Source: CAD feature listing. Evaluate the final solid. Frame: model axes, mm. A direction names the side the tool comes from. Round coordinates to 2 decimals unless told otherwise and drop trailing zeros. Write each loop counter-clockwise with the first axis right and the second up, starting at its lowest first coordinate (ties: lowest second). Pieces come first, ordered by that corner, then holes. Notation, with made-up numbers: M 21.5,31 L 67.5,31 A8 cw 67.5,46 Z; hole C 61.5,58 d2. An arc over 180 degrees is marked long. Answer in a Markdown table with one row per item.
from build123d import *

# Parameters (mm, degrees)
SKETCH1_W           = 43.699940619
SKETCH1_H           = 33.102984907
BOSS_EXTRUDE1_DEPTH = 10
BOSS_EXTRUDE2_DEPTH = 10
M3_TAPPED_HOLE1_D   = 4.2
SKETCH15_W          = 10
SKETCH15_H          = 17.102984907
SKETCH15_W_2        = 13
SKETCH15_H_2        = 47.102984907
CUT_EXTRUDE1_DEPTH  = 10
SKETCH18_W          = 58.662437665
SKETCH18_H          = 17.102984907
BOSS_EXTRUDE4_DEPTH = 10
BOSS_EXTRUDE5_DEPTH = 20
M8_TAPPED_HOLE2_D   = 6.8
FILLET1_R           = 5
FILLET2_R           = 1


with BuildPart() as part:
    # Sketch1 → Boss-Extrude1 (new body)
    with BuildSketch(Plane.XY):
        Polygon((42.979890311, 22.079670103), (-49.382487973, 22.079670103), (-49.382487973, -7.920329897), (-5.682547354, -7.920329897), (42.979890311, -7.920329897), align=None)
        with Locations((-27.532517664, -24.471822351)):
            Rectangle(SKETCH1_W, SKETCH1_H)
    extrude(amount=BOSS_EXTRUDE1_DEPTH)

    # Sketch10 → Boss-Extrude2 (add, symmetric)
    with BuildSketch(Plane(origin=(0, 7.079670103, 0), x_dir=(-1, 0, 0), z_dir=(0, -1, 0))):
        Polygon((-41.673127971, 0), (-24.707127971, 0), (-24.707127971, 2.991563555), align=None)
    extrude(amount=BOSS_EXTRUDE2_DEPTH, both=True)

    # M3 Tapped Hole1 (through all)
    with Locations(Plane(origin=(33.44592172, 6.992687386, -1.450678438), x_dir=(-0.984807753012, 0, -0.173648177667), z_dir=(0.173648177667, 0, -0.984807753012))):
        with Locations((0, 0)):
            Hole(M3_TAPPED_HOLE1_D / 2)

    # Sketch15 → Cut-Extrude1 (cut)
    with BuildSketch(Plane(origin=(0, 0, 0), x_dir=(-1, 0, 0), z_dir=(0, 0, -1))):
        Polygon((5.682547354, -25.023314804), (5.682547354, -41.023314804), (49.382487973, -41.023314804), (49.382487973, -25.023314804), (36.382487973, -25.023314804), (15.682547354, -25.023314804), align=None)
        with Locations((10.682547354, -16.471822351)):
            Rectangle(SKETCH15_W, SKETCH15_H)
        with Locations((42.882487973, -1.471822351)):
            Rectangle(SKETCH15_W_2, SKETCH15_H_2)
    extrude(amount=-CUT_EXTRUDE1_DEPTH, mode=Mode.SUBTRACT)

    # Sketch18 → Boss-Extrude4 (add)
    with BuildSketch(Plane(origin=(0, 0, 0), x_dir=(-1, 0, 0), z_dir=(0, 0, -1))):
        with Locations((-13.648671479, -16.471822351)):
            Rectangle(SKETCH18_W, SKETCH18_H)
    extrude(amount=-BOSS_EXTRUDE4_DEPTH)

    # Sketch19 → Boss-Extrude5 (add)
    with BuildSketch(Plane(origin=(0, 0, 0), x_dir=(-1, 0, 0), z_dir=(0, 0, -1))):
        with BuildLine():
            Line((36.382487973, -25.023314804), (15.730487973, -25.023314804))
            ThreePointArc((15.730487973, -25.023314804), (12.194954067, -23.55884871), (10.730487973, -20.023314804))
            Line((10.730487973, -20.023314804), (10.730487973, -4.371314804))
            ThreePointArc((10.730487973, -4.371314804), (12.194954067, -0.835780898), (15.730487973, 0.628685196))
            Line((15.730487973, 0.628685196), (31.382487973, 0.628685196))
            ThreePointArc((31.382487973, 0.628685196), (34.918021878, -0.835780898), (36.382487973, -4.371314804))
            Line((36.382487973, -4.371314804), (36.382487973, -25.023314804))
        make_face()
    extrude(amount=BOSS_EXTRUDE5_DEPTH)

    # M8 Tapped Hole2 (through all)
    with Locations(Plane(origin=(-28.692487973, -14.610329897, 10), x_dir=(1, 0, 0), z_dir=(0, 0, 1))):
        with Locations((0, 0)):
            Hole(M8_TAPPED_HOLE2_D / 2)

    # Fillet1
    fillet1_edges = [part.edges().sort_by_distance(p)[0] for p in [
        (-36.382487973, -25.023314804, -5),
        (-36.382487973, 22.079670103, 5),
        (42.979890311, -25.023314804, 5),
        (42.979890311, 22.079670103, 5),
    ]]
    fillet(fillet1_edges, radius=FILLET1_R)

    # Fillet2
    fillet2_edges = [part.edges().sort_by_distance(p)[0] for p in [
        (-36.382487973, -1.471822351, 10),
        (3.298701169, 22.079670103, 10),
        (3.298701169, -25.023314804, 10),
        (42.979890311, -1.471822351, 10),
        (-34.918021878, -23.55884871, 10),
        (41.515424217, -23.55884871, 10),
        (41.515424217, 20.615204009, 10),
        (-34.918021878, 20.615204009, 10),
    ]]
    fillet(fillet2_edges, radius=FILLET2_R)


solid = part.part
Q1. Section A-A (y = 11). Return loops of the section in (x, z), and give its area (3 significant figures).
Solutions:
| item | result |
|---|---|
| outline | M -36.38,0 L 24.71,0 L 24.71,-2.99 L 41.67,0 L 42.98,0 L 42.98,9 A1 ccw 41.98,10 L -35.38,10 A1 ccw -36.38,9 Z |
| area | 819 mm2 |
Q2. Contact query for flat-ended pins moving along their axis: pin 1 Ø3.5 at (y, z) = (3, -1.5) entering from -X; pin 2 Ø1.5 at (x, z) = (32, -1) entering from -Y; pin 3 Ø2 at (x, y) = (22, 7) entering from -Z; pin 4 Ø0.9 at (x, z) = (32, -1) entering from +Y. Output: stop coordinate, or through.
Solutions:
| item | result |
|---|---|
| pin 1 | stops at x = -36.38 |
| pin 2 | stops at y = -2.92 |
| pin 3 | stops at z = 0 |
| pin 4 | stops at y = 17.08 |
Q3. Material intervals for probe 1 along X at (y, z) = (-14.5, 5.25); probe 2 along X at (y, z) = (-7.5, -16.75); probe 3 along Z at (x, y) = (10, -20.5), sorted ascending.
Solutions:
| item | result |
|---|---|
| probe 1 | x = -36.38 to -32.09, -25.29 to 42.98 |
| probe 2 | x = -36.38 to -10.73 |
| probe 3 | z = 0 to 10 |
Q4. Section B-B (x = -30). Return loops of the section in (y, z).
Solutions:
| item | result |
|---|---|
| outline | M -25.02,-20 L -17.75,-20 L -17.75,10 L -24.02,10 A1 ccw -25.02,9 Z; M -11.47,-20 L 0.63,-20 L 0.63,0 L 22.08,0 L 22.08,9 A1 ccw 21.08,10 L -11.47,10 Z |
Q5. Section C-C (z = -11.75). Return loops of the section in (x, y), and give its area (3 significant figures).
Solutions:
| item | result |
|---|---|
| outline | M -36.38,-20.02 A5 ccw -31.38,-25.02 L -15.73,-25.02 A5 ccw -10.73,-20.02 L -10.73,-4.37 A5 ccw -15.73,0.63 L -31.38,0.63 A5 ccw -36.38,-4.37 Z; hole C -28.69,-14.61 d6.8 |
| area | 600 mm2 |
Q6. Section D-D (x = 7). Return loops of the section in (y, z).
Solutions:
| item | result |
|---|---|
| outline | M -25.02,0 L 22.08,0 L 22.08,9 A1 ccw 21.08,10 L -24.02,10 A1 ccw -25.02,9 Z |
Q7. Access query for faces 1 (the flat face through (-10.73, -12, -10)), 2 (the flat face through (24.707, 7, -1)), 3 (the flat face through (30, -2.92, -1)), 4 (the cylindrical face through (-34.88, -0.8, -9.86)). Directions: +Z, -Z, +X, -X, +Y, -Y. A direction counts if a zero-diameter tool reaches every point of the face in a straight line with its end or side. Return the directions, or none.
Solutions:
| item | result |
|---|---|
| face 1 | -Z, +X, +Y, -Y |
| face 2 | -Z, +Y, -Y |
| face 3 | -Z, +X, -Y |
| face 4 | -Z, -X, +Y |
